Can you work these out from the drawing? Everything is in mm from the part's minimum corner. A direction names the side the tool comes from. Round coordinates to 2 decimals unless told otherwise and drop trailing zeros. Order: outer loops, then holes, each group sorted by start corner. A loop starts at its lowest first (then second) coordinate and runs counter-clockwise, first axis right, second up. Notation, with made-up numbers: (62.5, 26.25) - (105.5, 26.25) arc R33 ccw to (105.5, 60.25) - close; hole circle Ø4 at (-19, 43.25). An arc over 180 degrees is marked (long way). Write item = value, one per line.
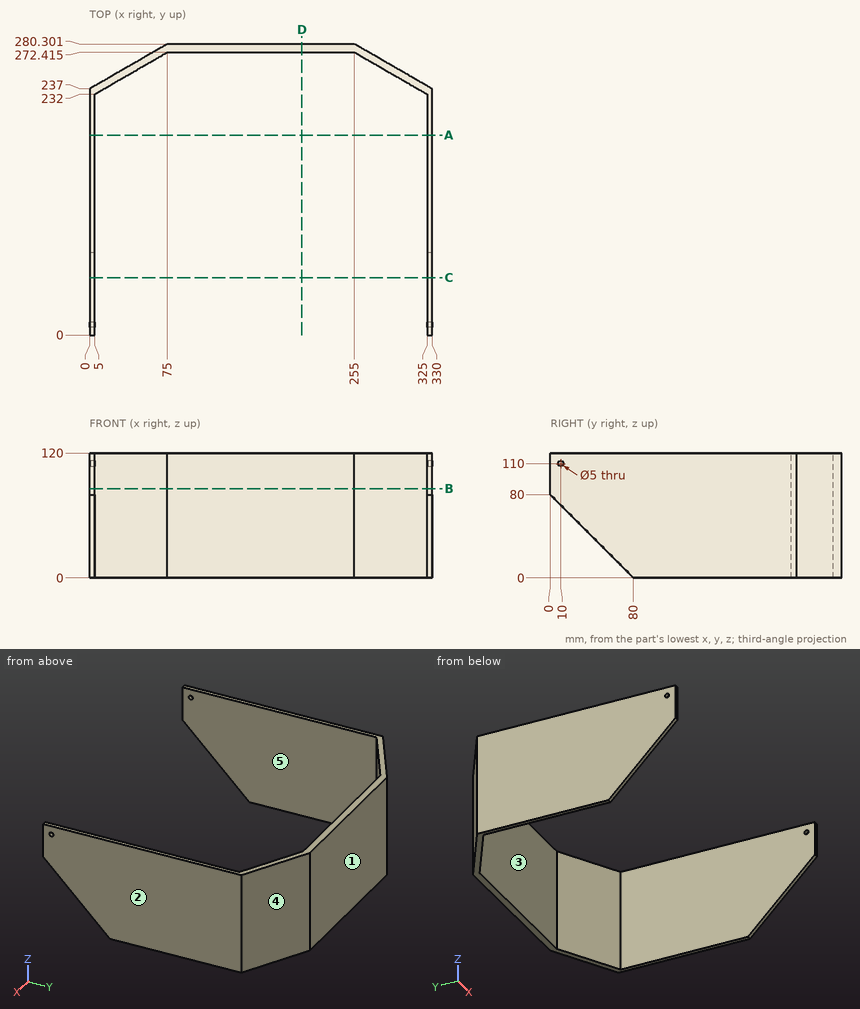
(1) If we section it at B-B (z = 86): Write out the boundary of the cut face in (x, y) (1 decimal).
Computed:
outline = (0, 0) - (5, 0) - (5, 232) - (75, 272.4) - (255, 272.4) - (325, 232) - (325, 0) - (330, 0) - (330, 237) - (255, 280.3) - (75, 280.3) - (0, 237) - close
(2) If we section it at D-D (x = 204.5): Write out the boundary of the cut face in (y, z) (1 decimal).
Computed:
outline = (272.4, 0) - (280.3, 0) - (280.3, 120) - (272.4, 120) - close
(3) On a 3-axis mill with a long thin cutter (end or side, diameter ignored), from which of +Z, -Z, +X, -X, +Y, -Y can I reach the whole of each face in a straight line? I mean the marked faces 4 and 5. Say none if no direction works.
Computed:
face_4 = +Z, -Z, +X, +Y
face_5 = +Z, -Z, -Y
(4) If we section it at A-A (y = 192.5): Write out the boundary of the cut face in (x, z).
Computed:
outline = (0, 0) - (5, 0) - (5, 120) - (0, 120) - close; (325, 0) - (330, 0) - (330, 120) - (325, 120) - close
(5) If I drill on line 1 (X direction, y = 214, z = 70.5); line 2 (Y direction, x = 86, z = 115) (1 decimal); line 3 (Y direction, x = 1, z = 110), over which ranges is the centre line in solid material (lowest first)? Write a range as from..to.
Computed:
line_1 = 0..5, 325..330
line_2 = 272.4..280.3
line_3 = 0..7.5, 12.5..237.58
(6) If we section it at C-C (y = 55.5): Write out the boundary of the cut face in (x, z).
Computed:
outline = (0, 24.5) - (5, 24.5) - (5, 120) - (0, 120) - close; (325, 24.5) - (330, 24.5) - (330, 120) - (325, 120) - close
(7) Thinking about a two-plate mould opening in X: for the marked faces 1, 2 and 3, which applies, +X half, -X half, draft (parallel to the pull), parting line (faces both ways), or undercut?
Computed:
face_1 = draft
face_2 = +X half
face_3 = undercut
(8) Will these pins go through, and if not, where does the flat tip stop? P1, Ø2, axis at x = 288.5, z = 12.5, coming from the +Y side; P2, Ø10, axis at x = 48, z = 18, coming from the -Y side; P3, Ø12, axis at x = 276, z = 105.5, coming from the -Y side (1 decimal).
Computed:
P1 = 261.54
P2 = 253.94
P3 = 256.8
